For this review, take the finished solid that the model builds, in its own axes (mm). A direction names the side the tool comes from. Give positions to 0.01 mm unless a question says otherwise; leave off trailing zeros. Loops run counter-clockwise (first coordinate to the right, second up) from the corner with the lowest first, then second, coordinate; pieces in that order, holes last.
```python
from build123d import *

# Parameters (mm, degrees)
BOSS_EXTRUDE1_DEPTH = 50
SKETCH2_W           = 100
SKETCH2_H           = 50
BOSS_EXTRUDE2_DEPTH = 90
SKETCH3_W           = 100
SKETCH3_H           = 30
BOSS_EXTRUDE3_DEPTH = 150
BOSS_EXTRUDE4_DEPTH = 10
FILLET1_R           = 50
CUT_EXTRUDE1_DEPTH  = 171.018381359


with BuildPart() as part:
    # Sketch1 → Boss-Extrude1 (new body)
    with BuildSketch(Plane(origin=(0, 0, 0), x_dir=(1, 0, 0), z_dir=(0, 1, 0))):
        with BuildLine():
            Line((30, -62.5), (50, -62.5))
            Line((50, -62.5), (50, 62.5))
            Line((50, 62.5), (-50, 62.5))
            Line((-50, 62.5), (-50, -62.5))
            Line((-50, -62.5), (-30, -62.5))
            ThreePointArc((-30, -62.5), (0, -32.5), (30, -62.5))
        make_face()
    extrude(amount=BOSS_EXTRUDE1_DEPTH)

    # Sketch2 → Boss-Extrude2 (add)
    with BuildSketch(Plane(origin=(0, 0, 0), x_dir=(1, 0, 0), z_dir=(0, 1, 0))):
        with Locations((0, 37.5)):
            Rectangle(SKETCH2_W, SKETCH2_H)
    extrude(amount=BOSS_EXTRUDE2_DEPTH)

    # Sketch3 → Boss-Extrude3 (add)
    with BuildSketch(Plane(origin=(0, 0, 0), x_dir=(1, 0, 0), z_dir=(0, 1, 0))):
        with Locations((0, 47.5)):
            Rectangle(SKETCH3_W, SKETCH3_H)
    extrude(amount=BOSS_EXTRUDE3_DEPTH)

    # Sketch4 → Boss-Extrude4 (add, symmetric)
    with BuildSketch(Plane(origin=(0, 0, 0), x_dir=(0, 0, -1), z_dir=(1, 0, 0))):
        Polygon((12.5, 90), (-27.5, 50), (12.5, 50), align=None)
    extrude(amount=BOSS_EXTRUDE4_DEPTH, both=True)

    # Fillet1
    fillet1_edges = [part.edges().sort_by_distance(p)[0] for p in [
        (-50, 150, -47.5),
        (50, 150, -47.5),
    ]]
    fillet(fillet1_edges, radius=FILLET1_R - 0.0001)  # a hair under: the kernel refuses the full size

    # Sketch6 → Cut-Extrude1 (cut, through all)
    with BuildSketch(Plane.XY):
        with BuildLine():
            Line((-30, 100), (30, 100))
            ThreePointArc((30, 100), (0, 130), (-30, 100))
        make_face()
    extrude(amount=-CUT_EXTRUDE1_DEPTH, mode=Mode.SUBTRACT)


solid = part.part
```
Q1. For pin 1 Ø12 at (x, y) = (21.5, 66.5) entering from +Z; pin 2 Ø10 at (x, z) = (23.5, -27) entering from +Y; pin 3 Ø6 at (x, z) = (13.5, -48) entering from -Y; pin 4 Ø6 at (x, z) = (-13.5, -36.5) entering from +Y, all flat-tipped, find the tip position at first contact; note any pin that passes through.
Answers:
pin 1: stops at z = -12.5
pin 2: stops at y = 90
pin 3: stops at y = 0
pin 4: stops at y = 148.89
Q2. Mouldability with a two-part tool opening along Y and no side actions: class faces 4 (the flat face through (-50, 38, -15)), 5 (the flat face through (0, 100, -47)), 6 (the flat face through (-12, 50, 16)) as +Y half, -Y half, draft (parallel to the pull), parting line (faces both ways), or undercut.
Answers:
face 4: draft
face 5: undercut
face 6: +Y half
Q3. For probe 1 along X at (y, z) = (69.5, -7.5); probe 2 along Z at (x, y) = (-23, 83); probe 3 along Z at (x, y) = (-33.5, 112), list the stretches that pass through material, from the lowest coordinate up.
Answers:
probe 1: x = -10 to 10
probe 2: z = -62.5 to -12.5
probe 3: z = -62.5 to -32.5
Q4. Consider section C-C on x = -22. Give the boundary of the cut face in (y, z).
Answers:
outline: (0, -62.5) - (100, -62.5) - (100, -32.5) - (90, -32.5) - (90, -12.5) - (50, -12.5) - (50, 42.1) - (0, 42.1) - close; (120.4, -62.5) - (144.9, -62.5) - (144.9, -32.5) - (120.4, -32.5) - close
Q5. Consider section B-B on y = 86. Give the boundary of the cut face in (x, z), plus the area to 3 significant figures.
Answers:
outline: (-50, -62.5) - (50, -62.5) - (50, -12.5) - (10, -12.5) - (10, -8.5) - (-10, -8.5) - (-10, -12.5) - (-50, -12.5) - close
area: 5,080 mm2
Q6. Consider section D-D on y = 114.5. Give the boundary of the cut face in (x, z).
Answers:
outline: (-47.85, -62.5) - (-26.26, -62.5) - (-26.26, -32.5) - (-47.85, -32.5) - close; (26.26, -62.5) - (47.85, -62.5) - (47.85, -32.5) - (26.26, -32.5) - close
Q7. Machinability: for faces 1 (the flat face through (30, 70, -12.5)), 2 (the flat face through (-30, 70, -12.5)), 3 (the cylindrical face through (0.66, 129.993, -47.29)), which of the approach directions +Z, -Z, +X, -X, +Y, -Y give a long, thin tool a straight path to every point of the face, cutting with its end or side? Answer none if there is none.
Answers:
face 1: +Z, +X, +Y
face 2: +Z, -X, +Y
face 3: +Z, -Z
